Drawing for the job (mm, zero at the part's lowest x, y, z). Give positions to 0.01 mm unless a question says otherwise; leave off trailing zeros. Order: outer loops, then holes, each group sorted by start corner. A loop starts at its lowest first (then second) coordinate and runs counter-clockwise, first axis right, second up. Notation, with made-up numbers: (41.5, 77) -> (53.5, 77) arc R15 ccw to (53.5, 98) -> close; hole circle Ø2 at (-30.75, -2.75). An arc over 180 degrees is marked (long way). Use one line per item in the form item = value. Start each with the question number.
1) Cut at D-D, the plane x = 70.5. Give the cut face in (y, z), and give its area (3 significant figures).
2) Probe line 1 (Z direction, x = 50, y = 2); line 2 (X direction, y = 2.45, z = 50); line 3 (X direction, y = 1, z = 62.5). List the from-to ranges inside material, lowest first.
3) Cut at C-C, the plane y = 1.6. Give the cut face in (x, z).
4) Cut at A-A, the plane x = 50. Give the cut face in (y, z).
5) Cut at B-B, the plane z = 50. Give the cut face in (x, y).
6) Drop flat-ended pins along their axis: P1, Ø5, axis at x = 68, z = 23.5, coming from the -Y side; P2, Ø2.5, axis at x = 50, z = 56, coming from the -Y side; P3, Ø1.5, axis at x = 72.5, y = 2, coming from the +Z side; P4, Ø1.5, axis at y = 0.5, z = 84, coming from the -X side. Give the stop position or say it passes through.
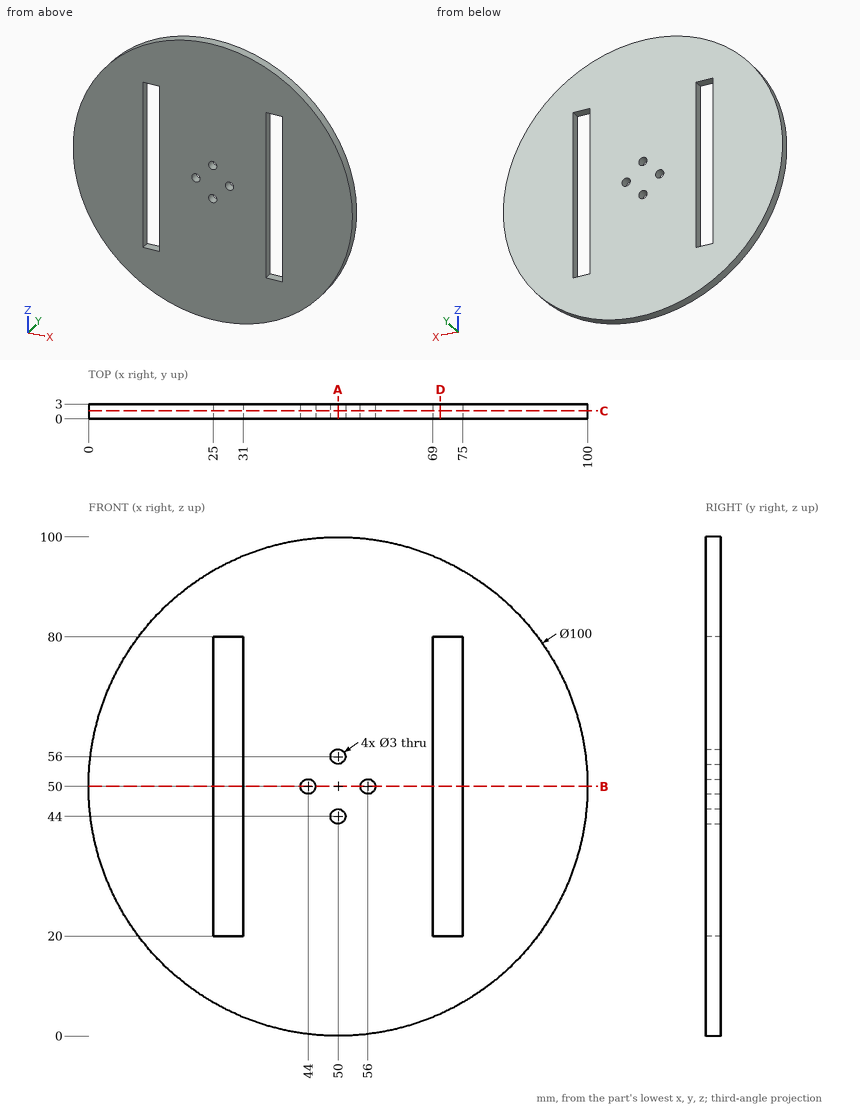
Result:
q1.outline = (0, 4.4) -> (3, 4.4) -> (3, 20) -> (0, 20) -> close; (0, 80) -> (3, 80) -> (3, 95.6) -> (0, 95.6) -> close
q1.area = 93.6 mm²
q2.line_1 = 0 to 42.5, 45.5 to 54.5, 57.5 to 100
q2.line_2 = 0 to 25, 31 to 42.5, 45.5 to 54.5, 57.5 to 69, 75 to 100
q2.line_3 = 1.59 to 25, 31 to 69, 75 to 98.41
q3.outline = circle Ø100 at (50, 50); hole (25, 20) -> (31, 20) -> (31, 80) -> (25, 80) -> close; hole circle Ø3 at (44, 50); hole circle Ø3 at (50, 44); hole circle Ø3 at (50, 56); hole circle Ø3 at (56, 50); hole (69, 20) -> (75, 20) -> (75, 80) -> (69, 80) -> close
q4.outline = (0, 0) -> (3, 0) -> (3, 42.5) -> (0, 42.5) -> close; (0, 45.5) -> (3, 45.5) -> (3, 54.5) -> (0, 54.5) -> close; (0, 57.5) -> (3, 57.5) -> (3, 100) -> (0, 100) -> close
q5.outline = (0, 0) -> (25, 0) -> (25, 3) -> (0, 3) -> close; (31, 0) -> (42.5, 0) -> (42.5, 3) -> (31, 3) -> close; (45.5, 0) -> (54.5, 0) -> (54.5, 3) -> (45.5, 3) -> close; (57.5, 0) -> (69, 0) -> (69, 3) -> (57.5, 3) -> close; (75, 0) -> (100, 0) -> (100, 3) -> (75, 3) -> close
q6.P1 = 0
q6.P2 = through
q6.P3 = 95.02
q6.P4 = 12.66
